Read the model definition and answer for the solid it produces. Units are mm, in the model's axes. Face numbers are marked on the shaded views. A direction names the side the tool comes from. Round coordinates to 2 decimals unless told otherwise and drop trailing zeros. Order: outer loops, then holes, each group sorted by start corner. A loop starts at its lowest first (then second) coordinate and runs counter-clockwise, first axis right, second up. Notation, with made-up numbers: (24, -29) -> (73, -29) arc R30 ccw to (73, -3) -> close; hole circle Ø10 at (-3.5, -25). An arc over 180 degrees is marked (long way). Use a Markdown table: item, result. Add a question column.
1. The mould has two halves that part along X. Classify the marked faces 1, 2, 3 and 4: +X half, -X half, draft (parallel to the pull), parting line (faces both ways), or undercut.
2. Section A-A, the plane x = -9 is taken. Give the vertices of the cut face in (y, z).
3. Section B-B, the plane y = 111.5 is taken. Give the vertices of the cut face in (x, z), then the cut area to 3 significant figures.
4. For the marked faces 5 and 6, determine the directions among +Z, -Z, +X, -X, +Y, -Y from which every point of the face is accessible in a straight line to the end or side of a thin tool.
5. Section C-C, the plane z = -3 is taken. Give the vertices of the cut face in (x, y).
6. Given pin 1 (1.5 mm diameter, centred on x = 28.5, y = 141, fed in from -Z); pin 2 (0.9 mm diameter, centred on y = 85, z = -28, fed in from +X); pin 3 (2.5 mm diameter, centred on x = 28, y = 138.5, fed in from +Z); pin 4 (8 mm diameter, centred on x = 3.5, z = -21.5, fed in from +Y), each flat-ended and moving along its own axis, determine where each tip first touches the part or whether it passes through.
7. Section D-D, the plane z = 16.5 is taken. Give the vertices of the cut face in (x, y), then the cut area to 3 significant figures.
8. Consider L1, parallel to Z at x = 6.5, y = 26; L2, parallel to Z at x = -22, y = 113. Determine where each line is inside the solid, lowest interval first. Write a range as [from, to].
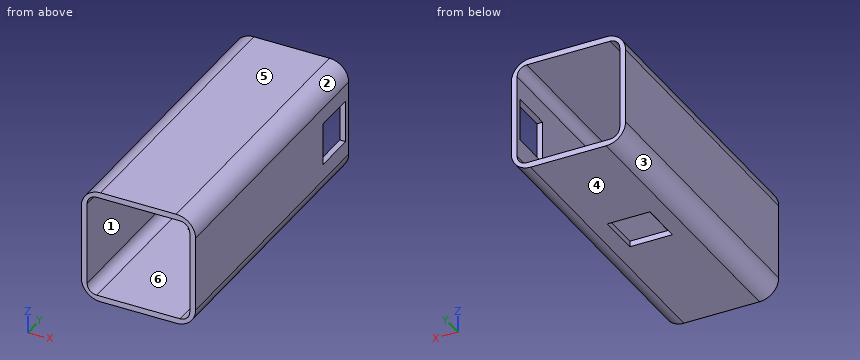
```python
from build123d import *

# Parameters (mm, degrees)
SKETCH1_W           = 59
SKETCH1_H           = 59
SKETCH1_W_2         = 53
SKETCH1_H_2         = 53
BOSS_EXTRUDE1_DEPTH = 150
FILLET1_R           = 10
FILLET2_R           = 5
SKETCH3_W           = 22
SKETCH3_H           = 22
CUT_EXTRUDE2_DEPTH  = 3
CUT_EXTRUDE4_REACH  = 165.864
SKETCH5_W           = 22
SKETCH5_H           = 22


with BuildPart() as part:
    # Sketch1 → Boss-Extrude1 (new body)
    with BuildSketch(Plane(origin=(0, 0, 0), x_dir=(1, 0, 0), z_dir=(0, 1, 0))):
        Rectangle(SKETCH1_W, SKETCH1_H)
        Rectangle(SKETCH1_W_2, SKETCH1_H_2, mode=Mode.SUBTRACT)
    extrude(amount=BOSS_EXTRUDE1_DEPTH)

    # Fillet1
    fillet1_edges = [part.edges().sort_by_distance(p)[0] for p in [
        (29.5, 75, 29.5),
        (-29.5, 75, 29.5),
        (-29.5, 75, -29.5),
        (29.5, 75, -29.5),
    ]]
    fillet(fillet1_edges, radius=FILLET1_R)

    # Fillet2
    fillet2_edges = [part.edges().sort_by_distance(p)[0] for p in [
        (26.5, 75, 26.5),
        (26.5, 75, -26.5),
        (-26.5, 75, -26.5),
        (-26.5, 75, 26.5),
    ]]
    fillet(fillet2_edges, radius=FILLET2_R)

    # Sketch3 → Cut-Extrude2 (cut)
    with BuildSketch(Plane(origin=(0, 0, -29.5), x_dir=(-1, 0, 0), z_dir=(0, 0, -1))):
        with Locations((0, 80)):
            Rectangle(SKETCH3_W, SKETCH3_H)
    extrude(amount=-CUT_EXTRUDE2_DEPTH, mode=Mode.SUBTRACT)

    # Sketch5 → Cut-Extrude4 (cut, up to next)
    with BuildSketch(Plane(origin=(29.5, 0, 0), x_dir=(0, 0, -1), z_dir=(1, 0, 0)), mode=Mode.PRIVATE) as cut_extrude4_sk1:
        with Locations((0, 136)):
            Rectangle(SKETCH5_W, SKETCH5_H)
    cut_extrude4_tool1 = extrude(cut_extrude4_sk1.sketch, amount=-CUT_EXTRUDE4_REACH, mode=Mode.PRIVATE) & part.part
    add(cut_extrude4_tool1.solids().sort_by_distance((29.5, 136, 0))[0], mode=Mode.SUBTRACT)


solid = part.part
```
Verdict:
| question | item | result |
|---|---|---|
| 1 | face 1 | undercut |
| 1 | face 2 | +X half |
| 1 | face 3 | -X half |
| 1 | face 4 | draft |
| 2 | outline | (0, -29.5) -> (69, -29.5) -> (69, -26.5) -> (0, -26.5) -> close; (0, 26.5) -> (150, 26.5) -> (150, 29.5) -> (0, 29.5) -> close; (91, -29.5) -> (150, -29.5) -> (150, -26.5) -> (91, -26.5) -> close |
| 3 | outline | (-29.5, -19.5) arc R10 ccw to (-19.5, -29.5) -> (19.5, -29.5) arc R10 ccw to (29.5, -19.5) -> (29.5, 19.5) arc R10 ccw to (19.5, 29.5) -> (-19.5, 29.5) arc R10 ccw to (-29.5, 19.5) -> close; hole (-26.5, -21.5) arc R5 ccw to (-21.5, -26.5) -> (21.5, -26.5) arc R5 ccw to (26.5, -21.5) -> (26.5, 21.5) arc R5 ccw to (21.5, 26.5) -> (-21.5, 26.5) arc R5 ccw to (-26.5, 21.5) -> close |
| 3 | area | 608 mm2 |
| 4 | face 5 | +Z, +X, -X, +Y, -Y |
| 4 | face 6 | +Y, -Y |
| 5 | outline | (-29.5, 0) -> (-26.5, 0) -> (-26.5, 150) -> (-29.5, 150) -> close; (26.5, 0) -> (29.5, 0) -> (29.5, 125) -> (26.5, 125) -> close; (26.5, 147) -> (29.5, 147) -> (29.5, 150) -> (26.5, 150) -> close |
| 6 | pin 1 | stops at z = -25.15 |
| 6 | pin 2 | stops at x = 25.43 |
| 6 | pin 3 | stops at z = 26.39 |
| 6 | pin 4 | passes through |
| 7 | outline | (-29.5, 0) -> (-26.5, 0) -> (-26.5, 150) -> (-29.5, 150) -> close; (26.5, 0) -> (29.5, 0) -> (29.5, 150) -> (26.5, 150) -> close |
| 7 | area | 900 mm2 |
| 8 | L1 | z = [-29.5, -26.5], [26.5, 29.5] |
| 8 | L2 | z = [-29.18, -26.47], [26.47, 29.18] |
